Part model, mm, in its own coordinate system. Give positions to 0.01 mm unless a question says otherwise; leave off trailing zeros. Write each loop counter-clockwise with the first axis right and the second up, starting at its lowest first coordinate (ties: lowest second). Pieces come first, ordered by that corner, then holes. Notation, with made-up numbers: M -8.5,43.5 L 16.5,43.5 A4 ccw 16.5,50.5 Z; hole C 42.25,-2.75 d7. An arc over 180 degrees is marked long. Answer as CSV lines item,"result". Start each with the question number.
Item 1: Two-plate mould, pull along Z, no slides. Class faces 1 (the flat face through (18.506, 1, 9)), 2 (the cylindrical face through (6.798, 1.288, 21.383)), 3 (the flat face through (6, 1, 24.584)): +Z half, -Z half, draft (parallel to the pull), parting line (faces both ways), or undercut.
Item 2: Band-saw the part on B-B, the plane x = 5. List the corners of the cut face in (y, z).
Item 3: Pin check, flat tip, straight feed: pin 1 (1.9 mm diameter, centred on x = 1.06, z = -0.82, fed in from +Y). Stop position of the tip, or through.
Item 4: Wall check: L1, parallel to Z at x = 1, y = 0.4; L2, parallel to Z at x = 7.5, y = 1.7; L3, parallel to X at y = 1.85, z = -0.5. Give the ranges that are in metal, low to high. Write a range as from..to.
Item 5: Band-saw the part on D-D, the plane y = 0.65. List the corners of the cut face in (x, z), then the cut area to 3 significant figures.
Item 6: Band-saw the part on A-A, the plane z = 0. List the corners of the cut face in (x, y), then the cut area to 3 significant figures.
Item 7: Band-saw the part on C-C, the plane z = 18. List the corners of the cut face in (x, y).
from build123d import *

# Parameters (mm, degrees)
SKETCH2_W                  = 25.4
SKETCH2_H                  = 31.75
BOSS_EXTRUDE1_DEPTH        = 2.54
F_2_4_2_4_DIAMETER_SLOT2_D = 2.4
SKETCH10_R                 = 3.302
CUT_EXTRUDE1_DEPTH         = 3.175


with BuildPart() as part:
    # Sketch2 → Boss-Extrude1 (new body)
    with BuildSketch(Plane(origin=(0, 0, 0), x_dir=(1, 0, 0), z_dir=(0, 1, 0))):
        with Locations((5.805714286, -8.708571429)):
            Rectangle(SKETCH2_W, SKETCH2_H)
    extrude(amount=BOSS_EXTRUDE1_DEPTH)

    # Ø2.4 (2.4) Diameter Slot2 (through all)
    with Locations(Plane(origin=(0, 2.54, 0), x_dir=(1, 0, 0), z_dir=(0, 1, 0))):
        with Locations((1.055714286, 0.816428571), (10.555714286, 0.816428571)):
            Hole(F_2_4_2_4_DIAMETER_SLOT2_D / 2)

    # Sketch10 → Cut-Extrude1 (cut)
    with BuildSketch(Plane(origin=(0, 2.54, 0), x_dir=(1, 0, 0), z_dir=(0, 1, 0))):
        with Locations(Location((5.805714286, -18.233571429, 0), (0, 0, 270))):
            Circle(SKETCH10_R)
    extrude(amount=-CUT_EXTRUDE1_DEPTH, mode=Mode.SUBTRACT)


solid = part.part
Output:
1,face 1,"draft"
1,face 2,"undercut"
1,face 3,"+Z half"
2,outline,"M 0,-7.17 L 2.54,-7.17 L 2.54,15.03 L 0,15.03 Z; M 0,21.44 L 2.54,21.44 L 2.54,24.58 L 0,24.58 Z"
3,pin 1,"through"
4,L1,"-7.17..-2.02, 0.38..24.58"
4,L2,"-7.17..15.4, 21.07..24.58"
4,L3,"-6.89..-0.1, 2.21..9.4, 11.71..18.51"
5,outline,"M -6.89,-7.17 L 18.51,-7.17 L 18.51,24.58 L -6.89,24.58 Z; hole C 1.06,-0.82 d2.4; hole C 5.81,18.23 d6.6; hole C 10.56,-0.82 d2.4"
5,area,"763 mm²"
6,outline,"M -6.89,0 L 0.18,0 L 0.18,2.54 L -6.89,2.54 Z; M 1.94,0 L 9.68,0 L 9.68,2.54 L 1.94,2.54 Z; M 11.44,0 L 18.51,0 L 18.51,2.54 L 11.44,2.54 Z"
6,area,"55.6 mm²"
7,outline,"M -6.89,0 L 2.51,0 L 2.51,2.54 L -6.89,2.54 Z; M 9.1,0 L 18.51,0 L 18.51,2.54 L 9.1,2.54 Z"
